from build123d import *

# Parameters (mm, degrees)
F0_R     = 5
F1_DEPTH = 10


with BuildPart() as f1:
    # F0 (on Front) → F1 (new body)
    with BuildSketch(Plane.XZ):
        Polygon((-25, 10), (-25, 0), (-25, -10), (-40, -10), (-40, -30), (-10, -30), (-10, -15), (0, -15), (10, -15), (10, -30), (40, -30), (40, -10), (25, -10), (25, 0), (25, 10), (40, 10), (40, 30), (10, 30), (10, 15), (0, 15), (-10, 15), (-10, 30), (-40, 30), (-40, 10), align=None)
        Circle(F0_R, mode=Mode.SUBTRACT)
    extrude(amount=F1_DEPTH)


solid = f1.part
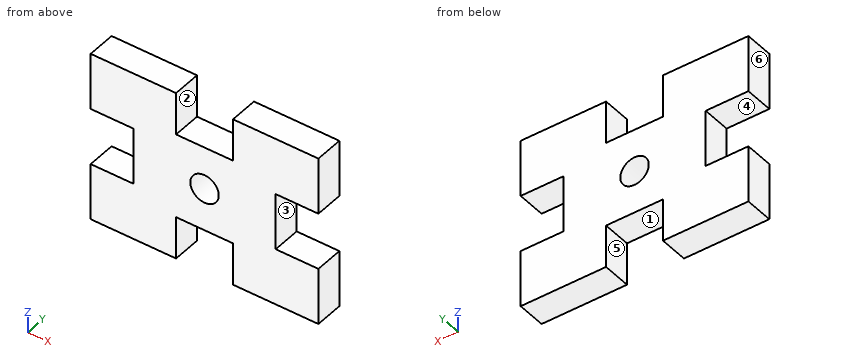
Model file for the job. Use its own axes, mm. Face numbers are marked on the shaded views. A direction names the side the tool comes from. Round coordinates to 2 decimals unless told otherwise and drop trailing zeros. Loops run counter-clockwise (first coordinate to the right, second up) from the corner with the lowest first, then second, coordinate; pieces in that order, holes last. Notation, with made-up numbers: (86.5, 47.5) - (126.5, 47.5) arc R23 ccw to (126.5, 76.5) - close; hole circle Ø8 at (10.25, 6). An arc over 180 degrees is marked (long way). Write each question's results on one line, items separated by ' | '.
(1) Saw through at B-B, the plane x = 3. List the corners of the cut face in (y, z), then the cut area to 3 significant figures.
Answer below:
outline: (-10, -15) - (0, -15) - (0, -4) - (-10, -4) - close; (-10, 4) - (0, 4) - (0, 15) - (-10, 15) - close | area: 220 mm^2
(2) 3-axis set-ups, long thin cutter, end or side, ignore diameter. For the marked faces 1, 2 and 3: which of +Z, -Z, +X, -X, +Y, -Y reach the whole face in a straight line?
Answer below:
face 1: -Z, +Y, -Y | face 2: +Z, +Y, -Y | face 3: +X, +Y, -Y
(3) Pin check, flat tips, straight feed: pin 1 (5 mm diameter, centred on x = 2.5, y = -3, fed in from +Z); pin 2 (2 mm diameter, centred on y = -2, z = 7, fed in from -X); pin 3 (5 mm diameter, centred on x = -0.5, y = -4, fed in from -Z); pin 4 (2 mm diameter, centred on x = 8, z = 21.5, fed in from -Y). Stop position of each tip, or through.
Answer below:
pin 1: stops at z = 15 | pin 2: stops at x = -25 | pin 3: stops at z = -15 | pin 4: passes through
(4) Wall check: L1, parallel to Z at x = -36, y = -2.5; L2, parallel to X at y = -2.5, z = -27; L3, parallel to Z at x = 0, y = -3.5. Give the ranges that are in metal, low to high.
Answer below:
L1: z = -30 to -10, 10 to 30 | L2: x = -40 to -10, 10 to 40 | L3: z = -15 to -5, 5 to 15
(5) Saw through at A-A, the plane z = 19. List the corners of the cut face in (x, y), then the cut area to 3 significant figures.
Answer below:
outline: (-40, -10) - (-10, -10) - (-10, 0) - (-40, 0) - close; (10, -10) - (40, -10) - (40, 0) - (10, 0) - close | area: 600 mm^2
(6) Saw through at C-C, the plane y = -5. List the corners of the cut face in (x, z), then the cut area to 3 significant figures.
Answer below:
outline: (-40, -30) - (-10, -30) - (-10, -15) - (10, -15) - (10, -30) - (40, -30) - (40, -10) - (25, -10) - (25, 10) - (40, 10) - (40, 30) - (10, 30) - (10, 15) - (-10, 15) - (-10, 30) - (-40, 30) - (-40, 10) - (-25, 10) - (-25, -10) - (-40, -10) - close; hole circle Ø10 at (0, 0) | area: 3,520 mm^2
(7) Mould opens along X. For the marked faces 4, 5 and 6 say: released by +X, released by -X, zero draft, split by the parting line, or undercut.
Answer below:
face 4: zero draft | face 5: undercut | face 6: released by -X
(8) Saw through at D-D, the plane x = -8. List the corners of the cut face in (y, z).
Answer below:
outline: (-10, -15) - (0, -15) - (0, 15) - (-10, 15) - close
